```python
from build123d import *

# Parameters (mm, degrees)
BOSS_EXTRUDE1_OUTLINE_R = 10
BOSS_EXTRUDE1_DEPTH     = 12
SKETCH5_R               = 6
BOSS_EXTRUDE2_DEPTH     = 20
CUT_EXTRUDE1_DEPTH      = 25.494897428


# Read off the part's stored shape, not the designer's step: Boss-Extrude1
with BuildPart() as part:
    # Boss-Extrude1 outline → Boss-Extrude1 (new body)
    with BuildSketch(Plane(origin=(0, 0, 0), x_dir=(0, 0, -1), z_dir=(1, 0, 0))):
        Circle(BOSS_EXTRUDE1_OUTLINE_R)
    extrude(amount=BOSS_EXTRUDE1_DEPTH)

    # Sketch5 → Boss-Extrude2 (add)
    with BuildSketch(Plane(origin=(12, 0, 0), x_dir=(0, 0, -1), z_dir=(1, 0, 0))):
        Circle(SKETCH5_R)
    extrude(amount=BOSS_EXTRUDE2_DEPTH)

    # Sketch7 → Cut-Extrude1 (cut, through all)
    with BuildSketch(Plane(origin=(12, 0, 0), x_dir=(0, 0, -1), z_dir=(1, 0, 0))):
        with BuildLine():
            Line((0, 7.797958971), (2, 7.797958971))
            Line((2, 7.797958971), (2, 9.797958971))
            ThreePointArc((2, 9.797958971), (0, 10), (-2, 9.797958971))
            Line((-2, 9.797958971), (-2, 7.797958971))
            Line((-2, 7.797958971), (0, 7.797958971))
        make_face()
    extrude(amount=-CUT_EXTRUDE1_DEPTH, mode=Mode.SUBTRACT)


solid = part.part
```
The model under review builds one solid part; all positions refer to its coordinate system, in mm. A direction names the side the tool comes from. Give positions to 0.01 mm unless a question says otherwise; leave off trailing zeros. Write each loop counter-clockwise with the first axis right and the second up, starting at its lowest first coordinate (ties: lowest second). Pieces come first, ordered by that corner, then holes.
(1) Consider section C-C, the plane x = 14. Give the boundary of the cut face in (y, z), and give its area (3 significant figures).
(2) Consider section A-A, the plane y = 0. Give the boundary of the cut face in (x, z), and give its area (3 significant figures).
(3) Consider section D-D, the plane z = -7.75. Give the boundary of the cut face in (x, y).
(4) Tool access review of faces 1 (the flat face through (0, 0, 0)), 2 (the flat face through (12, -4.4, -4.3)), 3 (the flat face through (6, 9, -2)): name each direction out of +Z, -Z, +X, -X, +Y, -Y from which nothing blocks a thin tool from reaching the whole face with its end or side.
(5) To check wall thickness, follow L1, parallel to X at y = 9, z = 3.75; L2, parallel to Y at x = 23.5, z = -4; L3, parallel to Z at x = 6.5, y = -3. State the ranges of each line that lie inside material, in increasing order.
(6) Consider section B-B, the plane z = 0. Give the boundary of the cut face in (x, y).
(7) For P1, Ø0.6, axis at x = 6, y = 8.5, coming from the -Z side; P2, Ø8, axis at x = 22, y = -2.5, coming from the -Z side; P3, Ø1.5, axis at x = 23, y = 5.5, coming from the +Z side, all flat-tipped, find the tip position at first contact; note any pin that passes through.
Returned:
1. outline: circle Ø12 at (0, 0)
1. area: 113 mm2
2. outline: (0, -10) - (12, -10) - (12, -6) - (32, -6) - (32, 6) - (12, 6) - (12, 10) - (0, 10) - close
2. area: 480 mm2
3. outline: (0, -6.32) - (12, -6.32) - (12, 6.32) - (0, 6.32) - close
4. face 1: +Z, -Z, -X, +Y, -Y
4. face 2: +X
4. face 3: +X, -X, +Y
5. L1: x = 0 to 12
5. L2: y = -4.47 to 4.47
5. L3: z = -9.54 to 9.54
6. outline: (0, -10) - (12, -10) - (12, -6) - (32, -6) - (32, 6) - (12, 6) - (12, 7.8) - (0, 7.8) - close
7. P1: stops at z = -5.72
7. P2: stops at z = -6
7. P3: stops at z = 3.67
